```python
from build123d import *

# Parameters (mm, degrees)
F1_DEPTH = 5
F2_R     = 3.75
F3_DEPTH = 2
F4_D     = 3.5
F5_W     = 4.8
F5_H     = 6
F6_DEPTH = 1.5
F7_R     = 0.5


with BuildPart() as f1:
    # F0 (on Top) → F1 (new body)
    with BuildSketch(Plane.XY):
        Polygon((17, 29), (-17, 29), (-17, -27), (-5.5, -27), (5.5, -27), (17, -27), align=None)
        with BuildLine():
            Line((5.5, -27), (-5.5, -27))
            Line((-5.5, -27), (-5.5, -34))
            ThreePointArc((-5.5, -34), (0, -28.5), (5.5, -34))
            Line((5.5, -34), (5.5, -27))
        make_face()
        with BuildLine():
            ThreePointArc((5.5, -34), (0, -28.5), (-5.5, -34))
            ThreePointArc((-5.5, -34), (0, -39.5), (5.5, -34))
        make_face()
    extrude(amount=F1_DEPTH)

    # F2 (on face) → F3 (join)
    with BuildSketch(Plane.XY.offset(5)):
        with Locations((0, -34)):
            Circle(F2_R)
    extrude(amount=F3_DEPTH)

    # F4 (through all)
    with Locations(Plane(origin=(0, 0, 0), x_dir=(1, 0, 0), z_dir=(0, 0, -1))):
        with Locations((0, 34)):
            Hole(F4_D / 2)

    # F5 (on face) → F6 (join)
    with BuildSketch(Plane.XY.offset(5)):
        with Locations((-7.6, 29)):
            Rectangle(F5_W, F5_H)
        with Locations((7.6, 29)):
            Rectangle(F5_W, F5_H)
    extrude(amount=F6_DEPTH)

    # F7
    f7_edges = [f1.edges().sort_by_distance(p)[0] for p in [
        (7.6, 26, 6.5),
        (-7.6, 26, 6.5),
        (-7.6, 32, 6.5),
        (7.6, 32, 6.5),
        (0, 29, 0),
        (17, 29, 2.5),
        (17, 1, 0),
        (17, -27, 2.5),
        (5.5, -30.5, 0),
        (0, -39.5, 0),
        (-3.75, -34, 7),
        (11.25, -27, 0),
        (-11.25, -27, 0),
        (-17, 1, 0),
        (10, 32, 5.75),
        (5.2, 32, 5.75),
        (-5.2, 32, 5.75),
        (-10, 32, 5.75),
        (-7.6, 26, 5),
        (7.6, 26, 5),
        (5.2, 27.5, 5),
        (-10, 27.5, 5),
        (-5.2, 27.5, 5),
        (10, 27.5, 5),
        (-5.5, -30.5, 0),
    ]]
    fillet(f7_edges, radius=F7_R)


solid = f1.part
```
Input: part model. Units: mm. Frame: model coordinates. A direction names the side the tool comes from. Coordinates: 2 decimals unless noted, no trailing zeros. Order: outer loops, then holes, each group sorted by start corner. A loop starts at its lowest first (then second) coordinate and runs counter-clockwise, first axis right, second up. Notation, with made-up numbers: (77.25, 39.5) - (92.25, 39.5) arc R13 ccw to (92.25, 50.5) - close; hole circle Ø6 at (67.5, -8). An arc over 180 degrees is marked (long way). Put each result on its own line as item: value.
1. Reachability of faces 4 (the face through (-8, 31, 5)), 5 (the face through (-5.5, -30, 3)), 6 (the face through (10, 29, 6)), 7 (the face through (11, -27, 3)), 8 (the face through (-10, 29, 6)) from +Z, -Z, +X, -X, +Y, -Y: full face, straight path, thin tool, end or side. Return the list, or none.
Report:
face 4: -Z, +X, -X, +Y
face 5: +Z, -Z, -X, -Y
face 6: +Z, +X, +Y
face 7: +Z, -Z, +X, -Y
face 8: +Z, -X, +Y
2. Contact query for flat-ended pins moving along their axis: pin 1 Ø3 at (x, z) = (-7, 2) entering from +Y; pin 2 Ø3 at (x, z) = (9, 4.5) entering from -Y; pin 3 Ø10 at (x, y) = (-11.5, -10) entering from +Z. Output: stop coordinate, or through.
Report:
pin 1: stops at y = 29
pin 2: stops at y = -27
pin 3: stops at z = 5
3. Cut plane D-D on y = -29. Return the cut outline in (x, z).
Report:
outline: (-5.5, 0.5) arc R0.5 ccw to (-5, 0) - (5, 0) arc R0.5 ccw to (5.5, 0.5) - (5.5, 5) - (-5.5, 5) - close
4. Draft query along Y for faces 1 (the face through (-11, -27, 3)), 2 (the face through (-1.669, -34.526, 3.549)), 3 (the face through (-5.2, 29, 6)). Return one class per face: pulls with the +Y half, pulls with the -Y half, needs draft (parallel to the pull), parting line crosses it, or undercut.
Report:
face 1: pulls with the -Y half
face 2: undercut
face 3: needs draft
5. Cut plane C-C on x = -8.5. Return the cut outline in (y, z), then the cut area to 3 significant figures.
Report:
outline: (-27, 0.5) arc R0.5 ccw to (-26.5, 0) - (28.5, 0) arc R0.5 ccw to (29, 0.5) - (29, 5) - (32, 5) - (32, 6) arc R0.5 ccw to (31.5, 6.5) - (26.5, 6.5) arc R0.5 ccw to (26, 6) - (26, 5.5) arc R0.5 cw to (25.5, 5) - (-27, 5) - close
area: 289 mm2
6. Cut plane A-A on x = 0. Return the cut outline in (y, z), then the cut area to 3 significant figures.
Report:
outline: (-39.5, 0.5) arc R0.5 ccw to (-39, 0) - (-35.75, 0) - (-35.75, 7) - (-37.25, 7) arc R0.5 ccw to (-37.75, 6.5) - (-37.75, 5) - (-39.5, 5) - close; (-32.25, 0) - (28.5, 0) arc R0.5 ccw to (29, 0.5) - (29, 5) - (-30.25, 5) - (-30.25, 6.5) arc R0.5 ccw to (-30.75, 7) - (-32.25, 7) - close
area: 333 mm2
7. Line query: line 1 along Y through (x, z) = (0, 4); line 2 along X through (y, z) = (-34, 3.5); line 3 along Y through (x, z) = (14.5, 3). Output: solid intervals per line, ascending.
Report:
line 1: y = -39.5 to -35.75, -32.25 to 29
line 2: x = -5.5 to -1.75, 1.75 to 5.5
line 3: y = -27 to 29
8. Cut plane B-B on y = -11.5. Return the cut outline in (x, z), then the cut area to 3 significant figures.
Report:
outline: (-17, 0.5) arc R0.5 ccw to (-16.5, 0) - (16.5, 0) arc R0.5 ccw to (17, 0.5) - (17, 5) - (-17, 5) - close
area: 170 mm2
